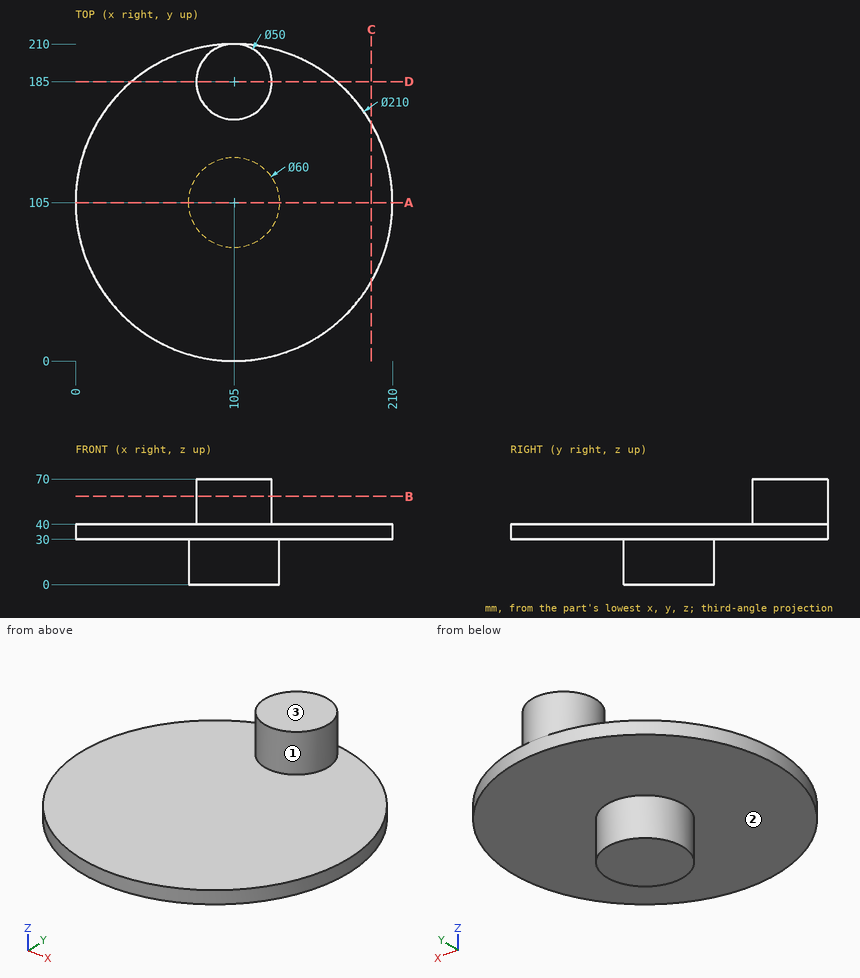
Design review of the part shown in the three views and the two pictorial views. Dimensions are in mm from the part's minimum x, y and z. A direction names the side the tool comes from. Round coordinates to 2 decimals unless told otherwise and drop trailing zeros. Loops run counter-clockwise (first coordinate to the right, second up) from the corner with the lowest first, then second, coordinate; pieces in that order, holes last. Notation, with made-up numbers: (7.5, 18.5) -> (11.5, 18.5) arc R22 cw to (11.5, 56.5) -> close; hole circle Ø1 at (-36.75, 85.5). An arc over 180 degrees is marked (long way). Return JSON: item names as keys, results as strings.
(1) Add section D-D on y = 185. Write out the cut boundary in (x, z).
Solved:
{"outline": "(36.99, 30) -> (173.01, 30) -> (173.01, 40) -> (130, 40) -> (130, 70) -> (80, 70) -> (80, 40) -> (36.99, 40) -> close"}
(2) For line 1 (Z direction, x = 148.5, y = 66); line 2 (Y direction, x = 106.5, z = 21.5); line 3 (Z direction, x = 122, y = 108), list the stretches that pass through material, from the lowest coordinate up.
Solved:
{"line 1": "30 to 40", "line 2": "75.04 to 134.96", "line 3": "0 to 40"}
(3) For pin 1 (2 mm diameter, centred on x = 36, y = 99.5, fed in from -Z); pin 2 (4 mm diameter, centred on y = 57.5, z = 31.5, fed in from +X); pin 3 (8 mm diameter, centred on x = 118, y = 66.5, fed in from +Z), all flat-tipped, find the tip position at first contact; note any pin that passes through.
Solved:
{"pin 1": "z = 30", "pin 2": "x = 199.63", "pin 3": "z = 40"}
(4) Add section B-B on z = 58.5. Write out the cut boundary in (x, y).
Solved:
{"outline": "circle Ø50 at (105, 185)"}
(5) For the marked faces 1, 2 and 3, list the 3-axis set-ups (+Z, -Z, +X, -X, +Y, -Y) from which the entire face can be reached by the end or side of a thin tool; tool diameter is ignored.
Solved:
{"face 1": "+Z", "face 2": "-Z", "face 3": "+Z, +X, -X, +Y, -Y"}
(6) Add section A-A on y = 105. Write out the cut boundary in (x, z), plus the area to 3 significant figures.
Solved:
{"outline": "(0, 30) -> (75, 30) -> (75, 0) -> (135, 0) -> (135, 30) -> (210, 30) -> (210, 40) -> (0, 40) -> close", "area": "3,900 mm2"}
(7) Add section C-C on x = 196. Write out the cut boundary in (y, z).
Solved:
{"outline": "(52.62, 30) -> (157.38, 30) -> (157.38, 40) -> (52.62, 40) -> close"}
